Model file for the job. Use its own axes, mm. A direction names the side the tool comes from. Coordinates: 2 decimals unless noted, no trailing zeros. Order: outer loops, then holes, each group sorted by start corner. A loop starts at its lowest first (then second) coordinate and runs counter-clockwise, first axis right, second up. Notation, with made-up numbers: (52.25, -8) -> (91.25, -8) arc R24 cw to (91.25, 6) -> close; hole circle Ø8 at (69.5, -32.75). An arc over 180 degrees is marked (long way). Return JSON: item names as keys, results as strings. Group by question number.
1) Which spindle directions (+Z, -Z, +X, -X, +Y, -Y) get a long thin tool onto all of the face, cutting with end or side? Do faces 3 (the cylindrical face through (38.303, 5.535, 91.302)), 4 (the flat face through (39, 1, 41.492)). Say none if no direction does.
2) Probe line 1 (X direction, y = 6.7, z = 30); line 2 (X direction, y = 3.25, z = 10); line 3 (X direction, y = 1.5, z = 101). List the from-to ranges inside material, lowest first.
3) Cut at B-B (z = 65). Write the cut outline in (x, y), and give its area (3 significant figures).
4) Pull direction Z, two halves, no side cores. Call faces 1 (the flat face through (0, 1, 96.3)), 2 (the flat face through (75, 4, 56)): +Z half, -Z half, draft (parallel to the pull), parting line (faces both ways), or undercut.
5) Cut at A-A (z = 101.3). Write the cut outline in (x, y), and give its area (4 significant figures).
from build123d import *

# Parameters (mm, degrees)
SKETCH1_W           = 150
SKETCH1_H           = 110
SKETCH1_R           = 2.5
BOSS_EXTRUDE1_DEPTH = 8
SKETCH3_R           = 1.5
CUT_EXTRUDE1_DEPTH  = 8
SKETCH4_R           = 1.5
CUT_EXTRUDE2_DEPTH  = 8
SKETCH5_W           = 10
SKETCH5_H           = 10
CUT_EXTRUDE3_DEPTH  = 3


with BuildPart() as part:
    # Sketch1 → Boss-Extrude1 (new body)
    with BuildSketch(Plane(origin=(0, 0, 0), x_dir=(1, 0, 0), z_dir=(0, 1, 0))):
        with Locations((0, -55)):
            Rectangle(SKETCH1_W, SKETCH1_H)
        with Locations(Location((-10, -65, 0), (0, 0, 270))):
            Circle(SKETCH1_R, mode=Mode.SUBTRACT)
        with Locations(Location((10, -65, 0), (0, 0, 270))):
            Circle(SKETCH1_R, mode=Mode.SUBTRACT)
        with Locations(Location((-20, -10, 0), (0, 0, 270))):
            Circle(SKETCH1_R, mode=Mode.SUBTRACT)
        with Locations(Location((20, -10, 0), (0, 0, 90))):
            Circle(SKETCH1_R, mode=Mode.SUBTRACT)
    extrude(amount=BOSS_EXTRUDE1_DEPTH)

    # Sketch3 → Cut-Extrude1 (cut)
    with BuildSketch(Plane(origin=(0, 8, 0), x_dir=(1, 0, 0), z_dir=(0, 1, 0))):
        with Locations(Location((-18, -30, 0), (0, 0, 270))):
            Circle(SKETCH3_R)
        with Locations(Location((18, -30, 0), (0, 0, 90))):
            Circle(SKETCH3_R)
        with Locations(Location((0, -101.3, 0), (0, 0, 270))):
            Circle(SKETCH3_R)
    extrude(amount=-CUT_EXTRUDE1_DEPTH, mode=Mode.SUBTRACT)

    # Sketch4 → Cut-Extrude2 (cut)
    with BuildSketch(Plane(origin=(0, 8, 0), x_dir=(1, 0, 0), z_dir=(0, 1, 0))):
        with Locations(Location((39.215686275, -46.492464754, 0), (0, 0, 270))):
            Circle(SKETCH4_R)
        with Locations(Location((63.215686275, -46.492464754, 0), (0, 0, 270))):
            Circle(SKETCH4_R)
        with Locations(Location((39.215686275, -92.492464754, 0), (0, 0, 270))):
            Circle(SKETCH4_R)
        with Locations(Location((63.215686275, -92.492464754, 0), (0, 0, 270))):
            Circle(SKETCH4_R)
    extrude(amount=-CUT_EXTRUDE2_DEPTH, mode=Mode.SUBTRACT)

    # Sketch5 → Cut-Extrude3 (cut)
    with BuildSketch(Plane.XZ):
        with Locations((0, 101.3)):
            Rectangle(SKETCH5_W, SKETCH5_H)
        with Locations((39.215686275, 92.492464754)):
            Rectangle(SKETCH5_W, SKETCH5_H)
        with Locations((63.215686275, 92.492464754)):
            Rectangle(SKETCH5_W, SKETCH5_H)
        with Locations((63.215686275, 46.492464754)):
            Rectangle(SKETCH5_W, SKETCH5_H)
        with Locations((39.215686275, 46.492464754)):
            Rectangle(SKETCH5_W, SKETCH5_H)
        with Locations((-18, 30)):
            Rectangle(SKETCH5_W, SKETCH5_H)
        with Locations((18, 30)):
            Rectangle(SKETCH5_W, SKETCH5_H)
    extrude(amount=-CUT_EXTRUDE3_DEPTH, mode=Mode.SUBTRACT)


solid = part.part
Answers below:
{
 "1": {"face 3": "+Y, -Y", "face 4": "-Y"},
 "2": {"line 1": "x = -75 to -19.5, -16.5 to 16.5, 19.5 to 75", "line 2": "x = -75 to -22.5, -17.5 to 17.5, 22.5 to 75", "line 3": "x = -75 to -5, 5 to 75"},
 "3": {"outline": "(-75, 0) -> (-12.5, 0) -> (-12.5, 8) -> (-75, 8) -> close; (-7.5, 0) -> (7.5, 0) -> (7.5, 8) -> (-7.5, 8) -> close; (12.5, 0) -> (75, 0) -> (75, 8) -> (12.5, 8) -> close", "area": "1,120 mm^2"},
 "4": {"face 1": "undercut", "face 2": "draft"},
 "5": {"outline": "(-75, 0) -> (-5, 0) -> (-5, 3) -> (-1.5, 3) -> (-1.5, 8) -> (-75, 8) -> close; (1.5, 3) -> (5, 3) -> (5, 0) -> (75, 0) -> (75, 8) -> (1.5, 8) -> close", "area": "1,155 mm^2"}
}
